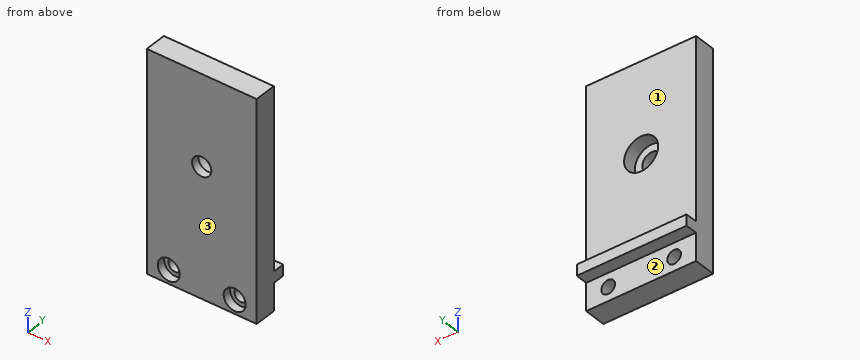
```python
from build123d import *

# Parameters (mm, degrees)
SKETCH_1_W          = 20
SKETCH_1_H          = 32.8
EXTRUDE_1_DEPTH     = 4
CUT_EXTRUDE_1_DEPTH = 1.6
SKETCH_4_R          = 2
CUT_EXTRUDE_2_DEPTH = 1.5
SKETCH_4_3_R        = 1.25
CUT_EXTRUDE_3_DEPTH = 39.624344655
SKETCH_5_W          = 20
SKETCH_5_H          = 6.2
EXTRUDE_4_DEPTH     = 2
EXTRUDE_START       = 2
SKETCH_5_6_W        = 20
SKETCH_5_6_H        = 4
EXTRUDE_5_DEPTH     = 5
SKETCH_6_R          = 1.25
CUT_EXTRUDE_4_DEPTH = 39.913750783
SKETCH_6_3_R        = 2
CUT_EXTRUDE_5_DEPTH = 1.5
SKETCH_1_3_W        = 20
SKETCH_1_3_H        = 32.8
EXTRUDE_6_DEPTH     = 4
SKETCH_7_R          = 3.1
CUT_EXTRUDE_7_DEPTH = 2.5
SKETCH_7_4_R        = 1.75
CUT_EXTRUDE_8_DEPTH = 39.624344655


with BuildPart() as part:
    # 草图1 → 凸台-拉伸1 (new body)
    with BuildSketch(Plane(origin=(0, 0, 0), x_dir=(1, 0, 0), z_dir=(0, 1, 0))):
        with Locations((10, -16.4)):
            Rectangle(SKETCH_1_W, SKETCH_1_H)
    extrude(amount=EXTRUDE_1_DEPTH)

    # 草图3 → 切除-拉伸1 (cut)
    with BuildSketch(Plane(origin=(0, 4, 0), x_dir=(-1, 0, 0), z_dir=(0, 1, 0))):
        with BuildLine():
            Line((-12.8, 13.543428629), (-12.095952788, 2.219685343))
            ThreePointArc((-12.095952788, 2.219685343), (-10, 0.25), (-7.904047212, 2.219685343))
            Line((-7.904047212, 2.219685343), (-7.2, 13.543428629))
            ThreePointArc((-7.2, 13.543428629), (-6, 16.4), (-7.2, 19.256571371))
            Line((-7.2, 19.256571371), (-7.904047212, 30.580314657))
            ThreePointArc((-7.904047212, 30.580314657), (-10, 32.55), (-12.095952788, 30.580314657))
            Line((-12.095952788, 30.580314657), (-12.8, 19.256571371))
            ThreePointArc((-12.8, 19.256571371), (-14, 16.4), (-12.8, 13.543428629))
        make_face()
    extrude(amount=-CUT_EXTRUDE_1_DEPTH, mode=Mode.SUBTRACT)

    # 草图4 → 切除-拉伸2 (cut)
    with BuildSketch(Plane.XZ):
        with Locations(Location((4, 4, 0), (0, 0, 270))):
            Circle(SKETCH_4_R)
        with Locations(Location((4, 28.8, 0), (0, 0, 270))):
            Circle(SKETCH_4_R)
        with Locations(Location((16, 28.8, 0), (0, 0, 270))):
            Circle(SKETCH_4_R)
        with Locations(Location((16, 4, 0), (0, 0, 270))):
            Circle(SKETCH_4_R)
    extrude(amount=-CUT_EXTRUDE_2_DEPTH, mode=Mode.SUBTRACT)

    # 草图4<3> → 切除-拉伸3 (cut, through all)
    with BuildSketch(Plane.XZ):
        with Locations(Location((4, 4, 0), (0, 0, 270))):
            Circle(SKETCH_4_3_R)
        with Locations(Location((4, 28.8, 0), (0, 0, 270))):
            Circle(SKETCH_4_3_R)
        with Locations(Location((16, 4, 0), (0, 0, 270))):
            Circle(SKETCH_4_3_R)
        with Locations(Location((16, 28.8, 0), (0, 0, 270))):
            Circle(SKETCH_4_3_R)
    extrude(amount=-CUT_EXTRUDE_3_DEPTH, mode=Mode.SUBTRACT)

    # 草图5 → 凸台-拉伸4 (add)
    with BuildSketch(Plane(origin=(0, 0, 0), x_dir=(-1, 0, 0), z_dir=(0, 0, -1))):
        with Locations((-10, 3.1)):
            Rectangle(SKETCH_5_W, SKETCH_5_H)
    extrude(amount=EXTRUDE_4_DEPTH)

    # 草图5<6> → 凸台-拉伸5 (add)
    with BuildSketch(Plane(origin=(0, 0, 0), x_dir=(-1, 0, 0), z_dir=(0, 0, -1)).offset(EXTRUDE_START)):
        with Locations((-10, 2)):
            Rectangle(SKETCH_5_6_W, SKETCH_5_6_H)
    extrude(amount=EXTRUDE_5_DEPTH)

    # 草图6 → 切除-拉伸4 (cut, through all)
    with BuildSketch(Plane.XZ):
        with Locations(Location((4, -4.5, 0), (0, 0, 270))):
            Circle(SKETCH_6_R)
        with Locations(Location((16, -4.5, 0), (0, 0, 270))):
            Circle(SKETCH_6_R)
    extrude(amount=-CUT_EXTRUDE_4_DEPTH, mode=Mode.SUBTRACT)

    # 草图6<3> → 切除-拉伸5 (cut)
    with BuildSketch(Plane.XZ):
        with Locations(Location((4, -4.5, 0), (0, 0, 270))):
            Circle(SKETCH_6_3_R)
        with Locations(Location((16, -4.5, 0), (0, 0, 270))):
            Circle(SKETCH_6_3_R)
    extrude(amount=-CUT_EXTRUDE_5_DEPTH, mode=Mode.SUBTRACT)

    # 草图1<3> → 凸台-拉伸6 (add)
    with BuildSketch(Plane(origin=(0, 0, 0), x_dir=(1, 0, 0), z_dir=(0, 1, 0))):
        with Locations((10, -16.4)):
            Rectangle(SKETCH_1_3_W, SKETCH_1_3_H)
    extrude(amount=EXTRUDE_6_DEPTH)

    # 草图7 → 切除-拉伸7 (cut)
    with BuildSketch(Plane(origin=(0, 4, 0), x_dir=(1, 0, 0), z_dir=(0, 1, 0))):
        with Locations(Location((10, -16.4, 0), (0, 0, 270))):
            Circle(SKETCH_7_R)
    extrude(amount=-CUT_EXTRUDE_7_DEPTH, mode=Mode.SUBTRACT)

    # 草图7<4> → 切除-拉伸8 (cut, through all)
    with BuildSketch(Plane(origin=(0, 4, 0), x_dir=(1, 0, 0), z_dir=(0, 1, 0))):
        with Locations(Location((10, -16.4, 0), (0, 0, 270))):
            Circle(SKETCH_7_4_R)
    extrude(amount=-CUT_EXTRUDE_8_DEPTH, mode=Mode.SUBTRACT)


solid = part.part
```
Geometry check sheet. Reference: the model listing, model coordinates, mm. Face numbers are marked on the shaded views. A direction names the side the tool comes from. Give positions to 0.01 mm unless a question says otherwise; leave off trailing zeros. Order: outer loops, then holes, each group sorted by start corner. A loop starts at its lowest first (then second) coordinate and runs counter-clockwise, first axis right, second up. Notation, with made-up numbers: (78, 67.25) - (118, 67.25) arc R14 ccw to (118, 78.25) - close; hole circle Ø1 at (64, 53). An arc over 180 degrees is marked (long way). Write item = value, one per line. Start each with the question number.
1) Scan lines: L1, parallel to X at y = 2.7, z = -4.5; L2, parallel to X at y = 0.7, z = -4.5; L3, parallel to X at y = 2.3, z = 16.4. Record each from-to range of solid material in increasing order.
2) Access from +Z, -Z, +X, -X, +Y, -Y to the whole of each face (thin tool, end or side, straight path). Record for the marked faces 1, 2 and 3.
3) Section check A-A (x = 4). Enter the section's corners in (y, z), then the cut area to 3 significant figures.
4) Section check C-C (z = -4.5). Enter the section's corners in (x, y).
5) Section check B-B (y = 3.25). Enter the section's corners in (x, z).
6) Gauge pin test, flat ends, axial feed: pin 1 Ø1.2 at (x, z) = (15, -4.5) entering from -Y; pin 2 Ø5.5 at (x, z) = (12.5, -4.5) entering from +Y; pin 3 Ø10 at (x, z) = (10, 16.4) entering from +Y; pin 4 Ø3 at (x, z) = (10.5, 15.5) entering from +Y. Record the tip position at first contact, or that the pin passes through.
7) Section check D-D (z = 16.4). Enter the section's corners in (x, y), then the cut area to 4 significant figures.
Geometry check:
q1.L1 = 0 to 2.75, 5.25 to 14.75, 17.25 to 20
q1.L2 = 0 to 2, 6 to 14, 18 to 20
q1.L3 = 0 to 6.9, 13.1 to 20
q2.face_1 = +Z, +X, -X, +Y
q2.face_2 = -Z, +X, -X, +Y
q2.face_3 = +Z, -Z, +X, -X, -Y
q3.outline = (0, -7) - (4, -7) - (4, -5.75) - (1.5, -5.75) - (1.5, -6.5) - (0, -6.5) - close; (0, -2.5) - (1.5, -2.5) - (1.5, -3.25) - (4, -3.25) - (4, -2) - (6.2, -2) - (6.2, 0) - (4, 0) - (4, 32.8) - (0, 32.8) - close
q3.area = 151 mm2
q4.outline = (0, 0) - (2, 0) - (2, 1.5) - (2.75, 1.5) - (2.75, 4) - (0, 4) - close; (5.25, 1.5) - (6, 1.5) - (6, 0) - (14, 0) - (14, 1.5) - (14.75, 1.5) - (14.75, 4) - (5.25, 4) - close; (17.25, 1.5) - (18, 1.5) - (18, 0) - (20, 0) - (20, 4) - (17.25, 4) - close
q5.outline = (0, -7) - (20, -7) - (20, 32.8) - (0, 32.8) - close; hole circle Ø2.5 at (4, -4.5); hole circle Ø6.2 at (10, 16.4); hole circle Ø2.5 at (16, -4.5)
q6.pin_1 = 1.5
q6.pin_2 = 6.2
q6.pin_3 = 4
q6.pin_4 = 1.5
q7.outline = (0, 0) - (8.25, 0) - (8.25, 1.5) - (6.9, 1.5) - (6.9, 4) - (0, 4) - close; (11.75, 0) - (20, 0) - (20, 4) - (13.1, 4) - (13.1, 1.5) - (11.75, 1.5) - close
q7.area = 59.25 mm2
